The listing builds one solid part. Answer for the finished solid, in the listing's coordinates (mm). Face numbers are marked on the shaded views. A direction names the side the tool comes from. Coordinates: 2 decimals unless noted, no trailing zeros. Order: outer loops, then holes, each group sorted by start corner. A loop starts at its lowest first (then second) coordinate and runs counter-clockwise, first axis right, second up.
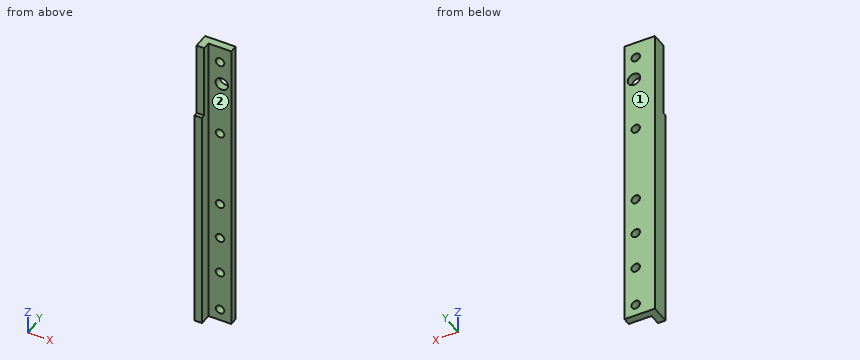
```python
from build123d import *

# Parameters (mm, degrees)
BOSS_EXTRUDE1_DEPTH  = 160
SKETCH2_W            = 39.551056564
SKETCH2_H            = 2
CUT_EXTRUDE1_DEPTH   = 4
M4_CLEARANCE_HOLE1_D = 4.5
SKETCH5_R            = 3.275
CUT_EXTRUDE2_DEPTH   = 10


with BuildPart() as part:
    # Sketch1 → Boss-Extrude1 (new body)
    with BuildSketch(Plane.XY):
        Polygon((0, 0), (0, -10), (4, -10), (4, -4), (16, -4), (16, 0), align=None)
    extrude(amount=BOSS_EXTRUDE1_DEPTH)

    # Sketch2 → Cut-Extrude1 (cut)
    with BuildSketch(Plane(origin=(4, 0, 0), x_dir=(0, 0, -1), z_dir=(1, 0, 0))):
        with Locations((-140.224471718, -9)):
            Rectangle(SKETCH2_W, SKETCH2_H)
    extrude(amount=-CUT_EXTRUDE1_DEPTH, mode=Mode.SUBTRACT)

    # M4 Clearance Hole1 (through all)
    with Locations(Plane(origin=(0, -4, 0), x_dir=(-1, 0, 0), z_dir=(0, -1, 0))):
        with Locations((-10.072352995, -6.228090532), (-10.072352995, -27.937872474), (-10.072352995, -48.221464361), (-10.072352995, -68.087621842), (-10.072352995, -109.517546491), (-10.072352995, -151.376567413)):
            Hole(M4_CLEARANCE_HOLE1_D / 2)

    # Sketch5 → Cut-Extrude2 (cut)
    with BuildSketch(Plane.XZ.offset(4)):
        with Locations(Location((11, 138.897931951, 0), (0, 0, 270))):
            Circle(SKETCH5_R)
    extrude(amount=-CUT_EXTRUDE2_DEPTH, mode=Mode.SUBTRACT)


solid = part.part
```
1) A cutting plane is placed at A-A, the plane z = 100. Write down the section's boundary in (x, y), plus the area to 3 significant figures.
2) Straight lines are drawn through the part: probe 1 along X at (y, z) = (-1.5, 138.5); probe 2 along Y at (x, z) = (14.5, 144); probe 3 along X at (y, z) = (-7.5, 68). For each, find the intervals that lie inside material, in ascending order.
3) Each of these flat-tipped pins is pushed along its axis until it touches: P1, Ø3, axis at x = 1.5, z = 138.5, coming from the -Y side; P2, Ø7.5, axis at x = 11, z = 138.9, coming from the -Y side; P3, Ø2, axis at y = -8.5, z = 33.5, coming from the +X side. Where does it stop, or does it pass through?
4) A cutting plane is placed at C-C, the plane y = -1.75. Write down the section's boundary in (x, z) (3 decimals), plus the area to 3 significant figures.
5) For the marked faces 1 and 2, determine the directions among +Z, -Z, +X, -X, +Y, -Y from which every point of the face is accessible in a straight line to the end or side of a thin tool.
6) A cutting plane is placed at B-B, the plane x = 11. Count the separate pieces of the cut face and the enclosed holes in it, plus the area to 3 significant figures.
Working result:
1. outline: (0, -10) - (4, -10) - (4, -4) - (16, -4) - (16, 0) - (0, 0) - close
1. area: 88.0 mm2
2. probe 1: x = 0 to 7.75, 14.25 to 16
2. probe 2: y = -4 to 0
2. probe 3: x = 0 to 4
3. P1: stops at y = -8
3. P2: stops at y = -4
3. P3: stops at x = 4
4. outline: (0, 0) - (16, 0) - (16, 160) - (0, 160) - close; hole circle Ø6.55 at (11, 138.898); hole circle Ø4.5 at (10.072, 6.228); hole circle Ø4.5 at (10.072, 27.938); hole circle Ø4.5 at (10.072, 48.221); hole circle Ø4.5 at (10.072, 68.088); hole circle Ø4.5 at (10.072, 109.518); hole circle Ø4.5 at (10.072, 151.377)
4. area: 2,430 mm2
5. face 1: +Z, -Z, +X, -X, +Y
5. face 2: +Z, -Z, +X, -Y
6. separate pieces: 8
6. enclosed holes: 0
6. area: 515 mm2
